Source: CAD feature listing. Evaluate the final solid. Frame: model axes, mm. Face numbers are marked on the shaded views. A direction names the side the tool comes from. Coordinates: 2 decimals unless noted, no trailing zeros. Loops run counter-clockwise (first coordinate to the right, second up) from the corner with the lowest first, then second, coordinate; pieces in that order, holes last.
Item 1: Pull-direction query (Y, two-part tool) for the marked faces 1, 2 and 3; classes: +Y half, -Y half, draft (parallel to the pull), parting line (faces both ways), or undercut.
Item 2: Line query: probe 1 along X at (y, z) = (-5.5, 0.75); probe 2 along X at (y, z) = (-1.5, 0.6); probe 3 along Y at (x, z) = (-52, 0.6). Output: solid intervals per line, ascending.
Item 3: Section query B-B, the plane y = -16. Return the cut outline in (x, z), then the cut area to 3 significant figures.
Item 4: Section query D-D, the plane y = -2. Return the cut outline in (x, z).
Item 5: Pin query (flat end, axial travel): pin 1 Ø0.9 at (y, z) = (-23.5, 1.5) entering from +X; pin 2 Ø12 at (x, y) = (-55, 10.5) entering from -Z; pin 3 Ø9 at (x, y) = (-39.5, -1) entering from +Z; pin 4 Ø1.5 at (x, z) = (-55.5, 1.5) entering from -Y. Return the tip coordinate at first contact, or that it passes through.
Item 6: Section query C-C, the plane x = -50. Return the cut outline in (y, z).
Item 7: Section query A-A, the plane z = 2.15. Return the cut outline in (x, y).
Item 8: Reachability of the marked faces 4 and 5 from +Z, -Z, +X, -X, +Y, -Y: full face, straight path, thin tool, end or side. Return the list, or none.
```python
from build123d import *

# Parameters (mm, degrees)
SALIENTE_EXTRUIR1_DEPTH = 3
CROQUIS2_R              = 9
CORTAR_EXTRUIR1_DEPTH   = 1.8
SALIENTE_EXTRUIR2_DEPTH = 1.2
SALIENTE_EXTRUIR3_DEPTH = 3
REDONDEO1_R             = 5


with BuildPart() as part:
    # Croquis1 → Saliente-Extruir1 (new body)
    with BuildSketch(Plane.XY):
        with BuildLine():
            Line((-39.310376575, -0.627009646), (-39.310376575, 19.872990354))
            ThreePointArc((-39.310376575, 19.872990354), (-14.810376575, -4.627009646), (-39.310376575, -29.127009646))
            Line((-39.310376575, -29.127009646), (-39.310376575, -8.627009646))
            ThreePointArc((-39.310376575, -8.627009646), (-35.310376575, -4.627009646), (-39.310376575, -0.627009646))
        make_face()
    extrude(amount=SALIENTE_EXTRUIR1_DEPTH)

    # Croquis2 → Cortar-Extruir1 (cut)
    with BuildSketch(Plane.XY.offset(3)):
        with Locations((-39.310376575, -4.627009646)):
            Circle(CROQUIS2_R)
    extrude(amount=-CORTAR_EXTRUIR1_DEPTH, mode=Mode.SUBTRACT)

    # Croquis3 → Saliente-Extruir2 (add)
    with BuildSketch(Plane.XY.offset(1.2)):
        with BuildLine():
            Line((-39.310376575, 4.372990354), (-39.310376575, -0.627009646))
            ThreePointArc((-39.310376575, -0.627009646), (-43.310376575, -4.627009646), (-39.310376575, -8.627009646))
            Line((-39.310376575, -8.627009646), (-39.310376575, -13.627009646))
            ThreePointArc((-39.310376575, -13.627009646), (-48.310376575, -4.627009646), (-39.310376575, 4.372990354))
        make_face()
    extrude(amount=-SALIENTE_EXTRUIR2_DEPTH)

    # Croquis4 → Saliente-Extruir3 (add)
    with BuildSketch(Plane.XY.offset(3)):
        with BuildLine():
            Line((-39.310376575, 19.872990354), (-39.310376575, 16.872990354))
            Line((-39.310376575, 16.872990354), (-43.310376575, 16.872990354))
            Line((-43.310376575, 16.872990354), (-43.310376575, 6.872990354))
            ThreePointArc((-43.310376575, 6.872990354), (-53.943204224, -4.627009646), (-43.310376575, -16.127009646))
            Line((-43.310376575, -16.127009646), (-43.310376575, -26.127009646))
            Line((-43.310376575, -26.127009646), (-39.310376575, -26.127009646))
            Line((-39.310376575, -26.127009646), (-39.310376575, -29.127009646))
            ThreePointArc((-39.310376575, -29.127009646), (-65.673236128, -4.627009646), (-39.310376575, 19.872990354))
        make_face()
    extrude(amount=-SALIENTE_EXTRUIR3_DEPTH)

    # Redondeo1
    redondeo1_edges = [part.edges().sort_by_distance(p)[0] for p in [
        (-43.310376575, 6.872990354, 1.5),
        (-43.310376575, -16.127009646, 1.5),
    ]]
    fillet(redondeo1_edges, radius=REDONDEO1_R)


solid = part.part
```
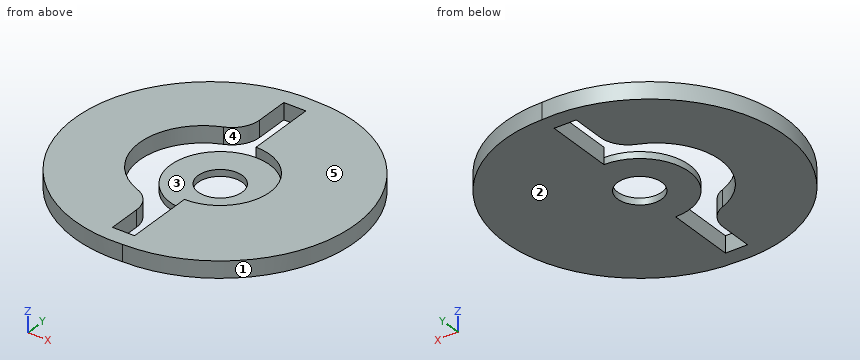
Verdict:
1. face 1: parting line
1. face 2: draft
1. face 3: undercut
2. probe 1: x = -65.66 to -53.91, -48.27 to -43.21, -35.41 to -14.83
2. probe 2: x = -65.47 to -53.51, -47.75 to -41.8, -36.82 to -15.01
2. probe 3: y = -26.65 to -11.03, 1.78 to 17.39
3. outline: (-62.88, 0) - (-45.41, 0) - (-45.41, 3) - (-62.88, 3) - close; (-39.31, 0) - (-17.61, 0) - (-17.61, 3) - (-39.31, 3) - close
3. area: 118 mm2
4. outline: (-65.53, 0) - (-53.64, 0) - (-53.64, 3) - (-65.53, 3) - close; (-47.92, 0) - (-42.33, 0) - (-42.33, 1.2) - (-47.92, 1.2) - close; (-36.29, 0) - (-14.95, 0) - (-14.95, 3) - (-30.7, 3) - (-30.7, 1.2) - (-36.29, 1.2) - close
5. pin 1: stops at x = -23.16
5. pin 2: stops at z = 0
5. pin 3: stops at z = 1.2
5. pin 4: stops at y = -25.06
6. outline: (-27.53, 0) - (-13.31, 0) - (-13.31, 3) - (-27.53, 3) - close; (4.06, 0) - (18.27, 0) - (18.27, 3) - (4.06, 3) - close
7. outline: (-39.31, -29.13) arc R24.5 ccw to (-39.31, 19.87) arc R24.57 ccw (long way) to start; hole (-46.53, -15.4) arc R5 cw to (-43.31, -20.07) - (-43.31, -26.13) - (-39.31, -26.13) - (-39.31, -13.63) arc R9 ccw to (-39.31, 4.37) - (-39.31, 16.87) - (-43.31, 16.87) - (-43.31, 10.82) arc R5 cw to (-46.53, 6.15) arc R11.54 ccw to start
8. face 4: +Z, -Z
8. face 5: +Z, +X, -X, +Y, -Y
